Work out the finished part from the listing and answer in its coordinate system (mm). Face numbers are marked on the shaded views. A direction names the side the tool comes from. Round coordinates to 2 decimals unless told otherwise and drop trailing zeros. Order: outer loops, then holes, each group sorted by start corner. A loop starts at its lowest first (then second) coordinate and runs counter-clockwise, first axis right, second up. Notation, with made-up numbers: (16, 60) - (54, 60) arc R18 cw to (54, 89) - close; hole circle Ø2 at (-9, 27.5). An arc over 180 degrees is marked (long way). Answer in a Markdown table with one row per item.
Autodesk Inventor part; units mm, degrees
ref_plane "YZ Plane" through (0, 0, 0) normal (1, 0, 0) x (0, 1, 0)
ref_plane "XZ Plane" through (0, 0, 0) normal (0, 1, 0) x (-1, 0, 0)
ref_plane "XY Plane" through (0, 0, 0) normal (0, 0, 1) x (1, 0, 0)
sketch "Sketch1" plane through (0, 0, 0) normal (1, 0, 0) x (0, 1, 0)
  arc A0 (-50.2663, 19.7308) -> (-50.2663, -19.7308) centre (0, 0) ccw
  line L0 (24.8197, 37.5) -> (-24.2023, 37.5)
  line L1 (-24.2023, -37.5) -> (24.8197, -37.5)
  arc A1 (0, 12.5) -> (0, -12.5) centre (0, 0) ccw
  circle A2 centre (0, -22.5) radius 5.5
  circle A3 centre (0, 22.5) radius 5.5
  arc A4 (-24.2023, 37.5) -> (-50.2663, 19.7308) centre (-24.2023, 9.5) ccw
  line L2 (-14, 0) -> (-38, 0)
  arc A5 (-50.2663, -19.7308) -> (-24.2023, -37.5) centre (-24.2023, -9.5) ccw
  arc A6 (-22.5167, 13) -> (-32.909, 19) centre (-27.7128, 16) ccw
  arc A7 (-32.909, -19) -> (-22.5167, -13) centre (-27.7128, -16) ccw
  arc A8 (-32.909, 19) -> (-32.909, -19) centre (0, 0) ccw
  arc A9 (36, 12.5) -> (43.4536, 29.1667) centre (36, 22.5) ccw
  arc A10 (43.4536, -29.1667) -> (36, -12.5) centre (36, -22.5) ccw
  line L3 (0, 12.5) -> (0, -12.5)
  arc A11 (3.9746, 26.3016) -> (3.6179, 25.7471) centre (24.8197, 12.5) ccw
  arc A12 (-0.1803, 12.4987) -> (0, 9.5026) centre (24.8197, 12.5) ccw
  arc A13 (24.8197, -37.5) -> (43.4536, -29.1667) centre (24.8197, -12.5) ccw
  arc A14 (0, -9.5026) -> (-0.1803, -12.4987) centre (24.8197, -12.5) ccw
  arc A15 (43.4536, 29.1667) -> (24.8197, 37.5) centre (24.8197, 12.5) ccw
  line L4 (0, 12.5) -> (36, 12.5)
  line L5 (0, -12.5) -> (36, -12.5)
  circle A16 centre (36, 22.5) radius 5.5
  circle A17 centre (36, -22.5) radius 5.5
  arc A18 (-22.5167, 13) -> (-22.5167, -13) centre (0, 0) ccw
  dimension "d21" = 11
  dimension "d12" = 20
  dimension "d19" = 25
  dimension "d22" = 11
  dimension "d23" = 11
  dimension "d24" = 36
  dimension "d25" = 32
  dimension "d26" = 6
extrude "Extrusion1" add sketch "Sketch1" along normal mid plane 10 contours A4 L0 A15 A9 L4 A1 L5 A10 A13 L1 A5 A0
properties part number "hw7"
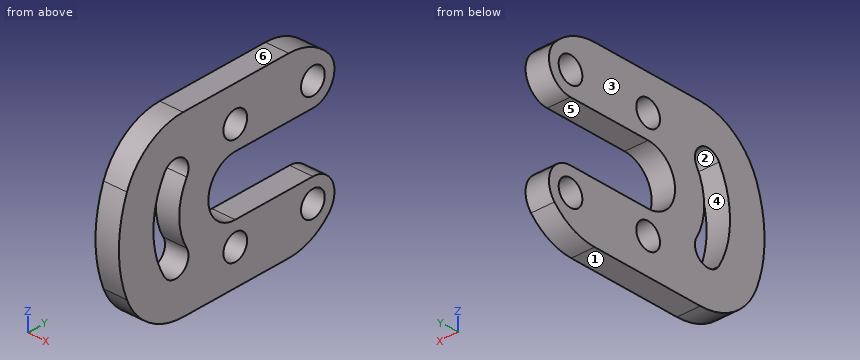
1) Which of the six approach directions +Z, -Z, +X, -X, +Y, -Y give full straight-line access (tool end or side, diameter ignored) to the marked faces 4, 5 and 6?
Filled in:
| item | result |
|---|---|
| face 4 | +X, -X |
| face 5 | +X, -X, +Y |
| face 6 | +Z, +X, -X, +Y, -Y |
2) Find section A-A, the plane y = 19.5. Give the vertices of the cut face in (x, z), then the cut area to 3 significant figures.
Filled in:
| item | result |
|---|---|
| outline | (-5, -37.5) - (5, -37.5) - (5, -12.5) - (-5, -12.5) - close; (-5, 12.5) - (5, 12.5) - (5, 37.5) - (-5, 37.5) - close |
| area | 500 mm^2 |
3) Find section B-B, the plane x = -0.75. Give the vertices of the cut face in (y, z).
Filled in:
| item | result |
|---|---|
| outline | (-50.27, -19.73) arc R28 ccw to (-24.2, -37.5) - (24.82, -37.5) arc R25 ccw to (43.45, -29.17) arc R10 ccw to (36, -12.5) - (0, -12.5) arc R12.5 cw to (0, 12.5) - (36, 12.5) arc R10 ccw to (43.45, 29.17) arc R25 ccw to (24.82, 37.5) - (-24.2, 37.5) arc R28 ccw to (-50.27, 19.73) arc R54 ccw to start; hole (-32.91, -19) arc R6 ccw to (-22.52, -13) arc R26 cw to (-22.52, 13) arc R6 ccw to (-32.91, 19) arc R38 ccw to start; hole circle Ø11 at (0, -22.5); hole circle Ø11 at (0, 22.5); hole circle Ø11 at (36, -22.5); hole circle Ø11 at (36, 22.5) |
4) Find the intervals of material crossed by probe 1 along Z at (x, y) = (3.25, 16); probe 2 along Z at (x, y) = (0.5, 36); probe 3 along Y at (x, z) = (-2, -25), in increasing order. Write a range as from..to.
Filled in:
| item | result |
|---|---|
| probe 1 | z = -37.5..-12.5, 12.5..37.5 |
| probe 2 | z = -34.86..-28, -17..-12.5, 12.5..17, 28..34.86 |
| probe 3 | y = -47.52..-4.9, 4.9..31.1, 40.9..45.68 |
5) Find section C-C, the plane z = 15. Give the vertices of the cut face in (x, y), then the cut area to 3 significant figures.
Filled in:
| item | result |
|---|---|
| outline | (-5, -51.87) - (5, -51.87) - (5, -34.91) - (-5, -34.91) - close; (-5, -21.8) - (5, -21.8) - (5, 42.61) - (-5, 42.61) - close |
| area | 814 mm^2 |
6) Each of these flat-tipped pins is pushed along its axis until it touches: pin 1 (1 mm diameter, centred on x = 1, z = -18, fed in from +Y); pin 2 (4 mm diameter, centred on x = -2, z = 8.5, fed in from -Y). Where does it stop, or does it pass through?
Filled in:
| item | result |
|---|---|
| pin 1 | stops at y = 45.17 |
| pin 2 | stops at y = -53.61 |
7) The mould has two halves that part along Z. Classify the marked faces 1, 2 and 3: released by +Z, released by -Z, zero draft, split by the parting line, or undercut.
Filled in:
| item | result |
|---|---|
| face 1 | released by -Z |
| face 2 | undercut |
| face 3 | zero draft |
